Autodesk Inventor part; units mm, degrees
ref_plane "YZ Plane" through (0, 0, 0) normal (1, 0, 0) x (0, 1, 0)
ref_plane "XZ Plane" through (0, 0, 0) normal (0, 1, 0) x (-1, 0, 0)
ref_plane "XY Plane" through (0, 0, 0) normal (0, 0, 1) x (1, 0, 0)
sketch "Sketch1" plane through (0, 0, 0) normal (0, 0, 1) x (1, 0, 0)
  circle A0 centre (0, 0) radius 12.5
  dimension "d0" = 25
extrude "Extrusion1" add sketch "Sketch1" along normal blind 228
sketch "Sketch2" plane through (0, 0, 0) normal (0, 1, 0) x (-1, 0, 0)
  line L0 (12.5, 228) -> (-12.5, 228)
  line L1 (-12.5, 0) -> (12.5, 0)
  line L2 (12.5, 0) -> (12.5, 228)
  line L3 (12.5, 228) -> (-12.5, 228)
  line L4 (12.5, 221.7204) -> (-12.5, 228)
  point P0 (0, 0)
  dimension "d5" = 14.1
extrude "Extrusion2" cut sketch "Sketch2" along normal through all both and the other way through all
sketch "Sketch3" plane through (0, 0, 0) normal (0, 1, 0) x (-1, 0, 0)
  line L0 (12.5, 0) -> (12.5, 221.7204)
  line L1 (-12.5, 0) -> (-12.5, 228)
  line L2 (-12.5, 0) -> (12.5, 0)
  line L3 (12.5, 2.953) -> (-12.5, 2.953)
  line L4 (-12.5, 2.953) -> (-12.5, 0)
  line L5 (-12.5, 0) -> (12.5, 0)
  line L6 (12.5, 0) -> (12.5, 2.953)
  point P0 (0, 0)
  dimension "d6" = 2.953
extrude "Extrusion3" cut sketch "Sketch3" along normal through all both and the other way through all
chamfer "Chamfer1" distance 3 angle 45 1 edges at (-12.5, 0, 2.953)
equation "\"d0\" = trappestifter_dia"
equation "\"d1\" = trappestifter_laengde"
equation "\"trappestifter_dia\" = 25"
equation "\"trappestifter_laengde\" = 228"
equation "\"perforeringsbredde\" = 6"
equation "\"perforeringshullaengde\" = 62.8"
equation "\"perforeringsoffset\" = 8"
equation "\"perforeringsoffset_top\" = 8"
equation "\"perforeringsoffset_bund\" = 8"
equation "\"laskehul_dia\" = 13"
equation "\"perforeringshullaengde_bund\" = 61.6"
equation "\"perforeringshullaengde_top\" = 61"
equation "\"trappestifter_huldia\" = 25.8"
equation "\"trappestifter_skraa_huldia\" = 26.6"
equation "\"trappevinkel\" = 34.3deg"
equation "\"balusterhul_udvidelse\" = 1"
equation "\"pladetykkelse\" = 3"
equation "\"trinbredde\" = 1884"
properties part number "trappestift skrå" material "S355J2"
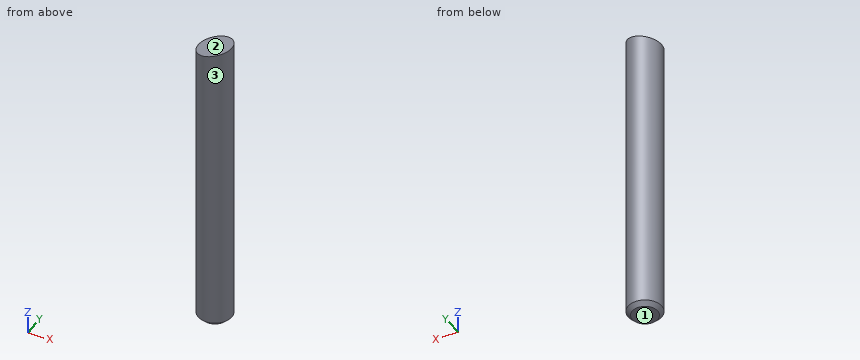
Geometry check sheet. Reference: the model listing, model coordinates, mm. Face numbers are marked on the shaded views. Give positions to 0.01 mm unless a question says otherwise; leave off trailing zeros. Write each loop counter-clockwise with the first axis right and the second up, starting at its lowest first coordinate (ties: lowest second). Pieces come first, ordered by that corner, then holes.
1) Section check B-B, the plane z = 72. Record the boundary of the cut face in (x, y).
2) Section check C-C, the plane x = 0. Record the boundary of the cut face in (y, z).
3) Material ranges on L1, parallel to Y at x = -0.25, z = 173.5; L2, parallel to Z at x = -4.5, y = -4.5; L3, parallel to X at y = 7, z = 81, recorded low to high.
4) Release check for a two-part mould opening along X. For the marked faces 1, 2 and 3 record: pulls with the +X half, pulls with the -X half, needs draft (parallel to the pull), parting line crosses it, or undercut.
5) Gauge pin test, flat ends, axial feed: pin 1 (1.5 mm diameter, centred on y = -5, z = 109, fed in from +X); pin 2 (6 mm diameter, centred on y = -3.5, z = 162.5, fed in from -X); pin 3 (8 mm diameter, centred on y = -6, z = 110.5, fed in from -X); pin 4 (8 mm diameter, centred on x = -9, y = -5, fed in from -Z). Record the tip position at first contact, or that the pin passes through.
6) Section check A-A, the plane y = 0. Record the boundary of the cut face in (x, z).
Computed:
1. outline: circle Ø25 at (0, 0)
2. outline: (-12.5, 5.95) - (-9.5, 2.95) - (9.5, 2.95) - (12.5, 5.95) - (12.5, 224.86) - (-12.5, 224.86) - close
3. L1: y = -12.5 to 12.5
3. L2: z = 2.95 to 223.73
3. L3: x = -10.36 to 10.36
4. face 1: needs draft
4. face 2: pulls with the -X half
4. face 3: parting line crosses it
5. pin 1: stops at x = 11.76
5. pin 2: stops at x = -12.49
5. pin 3: stops at x = -12.34
5. pin 4: stops at z = 2.95
6. outline: (-12.5, 5.95) - (-9.5, 2.95) - (9.5, 2.95) - (12.5, 5.95) - (12.5, 228) - (-12.5, 221.72) - close
